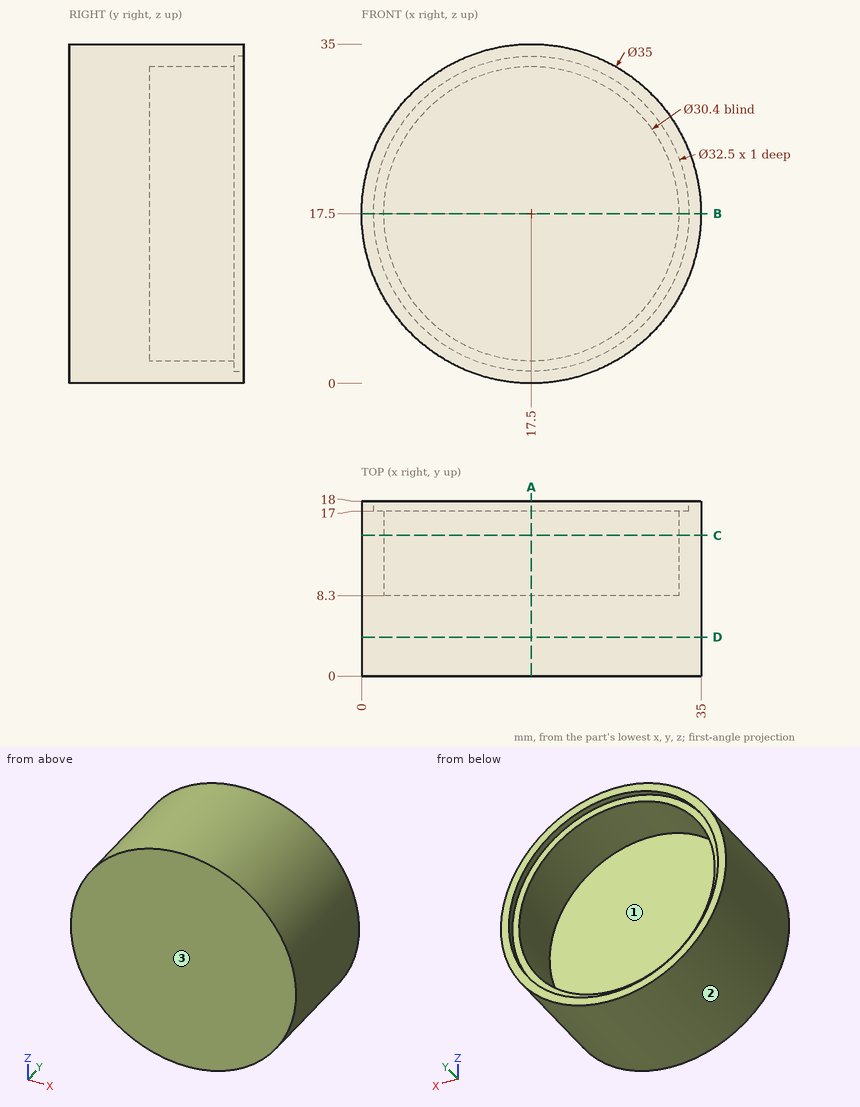
The figure shows three views and two pictorial views of one solid part (mm, origin at its lowest corner). Answer the questions. Give positions to 0.01 mm unless a question says otherwise; leave off trailing zeros. Order: outer loops, then holes, each group sorted by start corner. A loop starts at its lowest first (then second) coordinate and runs counter-clockwise, first axis right, second up. Notation, with made-up numbers: (37, 12.25) -> (58, 12.25) arc R26 cw to (58, 42.25) -> close; hole circle Ø1 at (5, 14.25). An arc over 180 degrees is marked (long way). Answer as a JSON object with one key per item and string values. Group by question number.
Item 1: The part is cut by section C-C on y = 14.5. Write down the section's boundary in (x, z).
Item 2: Determine the mould class of the marked faces 1, 2 and 3 for opening direction X: pulls with the +X half, pulls with the -X half, needs draft (parallel to the pull), parting line crosses it, or undercut.
Item 3: The part is cut by section B-B on z = 17.5. Write down the section's boundary in (x, y).
Item 4: The part is cut by section D-D on y = 4. Write down the section's boundary in (x, z), and give its area (3 significant figures).
Item 5: Flat-ended cylindrical pins translate along their axes: pin 1 (8 mm diameter, centred on y = 9.5, z = 26, fed in from -X); pin 2 (8 mm diameter, centred on y = 15.5, z = 6.5, fed in from +X); pin 3 (1.5 mm diameter, centred on x = 12.5, y = 2, fed in from -Z). Find the tip coordinate at first contact, or state that the pin passes through.
Item 6: The part is cut by section A-A on x = 17.5. Write down the section's boundary in (y, z), and give its area (3 significant figures).
Item 7: Consider L1, parallel to X at y = 12.75, z = 17.5; L2, parallel to Y at x = 21.5, z = 33; L3, parallel to Y at x = 28, z = 28. Determine where each line is inside the solid, lowest interval first. Write a range as from..to.
Result set:
{
 "1": {"outline": "circle Ø35 at (17.5, 17.5); hole circle Ø30.4 at (17.5, 17.5)"},
 "2": {"face 1": "undercut", "face 2": "parting line crosses it", "face 3": "needs draft"},
 "3": {"outline": "(0, 0) -> (35, 0) -> (35, 18) -> (33.75, 18) -> (33.75, 17) -> (32.7, 17) -> (32.7, 8.3) -> (2.3, 8.3) -> (2.3, 17) -> (1.25, 17) -> (1.25, 18) -> (0, 18) -> close"},
 "4": {"outline": "circle Ø35 at (17.5, 17.5)", "area": "962 mm²"},
 "5": {"pin 1": "x = 0.59", "pin 2": "x = 33.54", "pin 3": "z = 0.52"},
 "6": {"outline": "(0, 0) -> (18, 0) -> (18, 1.25) -> (17, 1.25) -> (17, 2.3) -> (8.3, 2.3) -> (8.3, 32.7) -> (17, 32.7) -> (17, 33.75) -> (18, 33.75) -> (18, 35) -> (0, 35) -> close", "area": "333 mm²"},
 "7": {"L1": "0..2.3, 32.7..35", "L2": "0..17", "L3": "0..8.3"}
}
